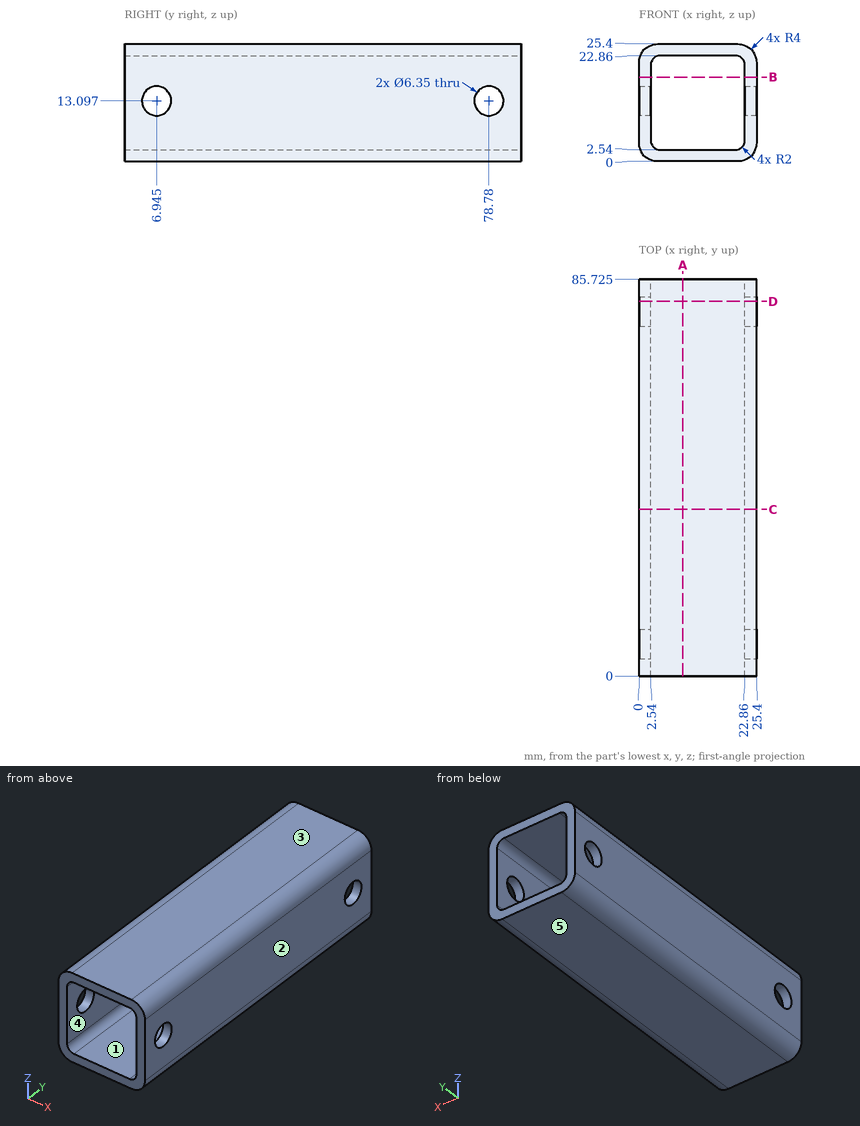
The drawing under review shows one solid part. Ordinate dimensions are in mm from its lowest x, y, z. A direction names the side the tool comes from. Round coordinates to 2 decimals unless told otherwise and drop trailing zeros. Write each loop counter-clockwise with the first axis right and the second up, starting at its lowest first coordinate (ties: lowest second). Pieces come first, ordered by that corner, then holes. Notation, with made-up numbers: (14, 12) -> (67, 12) arc R19 cw to (67, 27) -> close; hole circle Ø3 at (51, -8.5). An arc over 180 degrees is marked (long way). Put each result on its own line as item: value.
Q1. Machinability: for the marked faces 4 and 5, which of the approach directions +Z, -Z, +X, -X, +Y, -Y give a long, thin tool a straight path to every point of the face, cutting with its end or side? Answer none if there is none.
Determined:
face 4: +Y, -Y
face 5: -Z, +X, -X, +Y, -Y
Q2. Consider section D-D on y = 81. State the section outline as (x, z) points, and give its area (3 significant figures).
Determined:
outline: (0, 4) arc R4 ccw to (4, 0) -> (21.4, 0) arc R4 ccw to (25.4, 4) -> (25.4, 10.83) -> (22.86, 10.83) -> (22.86, 4.54) arc R2 cw to (20.86, 2.54) -> (4.54, 2.54) arc R2 cw to (2.54, 4.54) -> (2.54, 10.83) -> (0, 10.83) -> close; (0, 15.37) -> (2.54, 15.37) -> (2.54, 20.86) arc R2 cw to (4.54, 22.86) -> (20.86, 22.86) arc R2 cw to (22.86, 20.86) -> (22.86, 15.37) -> (25.4, 15.37) -> (25.4, 21.4) arc R4 ccw to (21.4, 25.4) -> (4, 25.4) arc R4 ccw to (0, 21.4) -> close
area: 199 mm^2
Q3. Consider section C-C on y = 36. State the section outline as (x, z) points, and give its area (3 significant figures).
Determined:
outline: (0, 4) arc R4 ccw to (4, 0) -> (21.4, 0) arc R4 ccw to (25.4, 4) -> (25.4, 21.4) arc R4 ccw to (21.4, 25.4) -> (4, 25.4) arc R4 ccw to (0, 21.4) -> close; hole (2.54, 4.54) arc R2 ccw to (4.54, 2.54) -> (20.86, 2.54) arc R2 ccw to (22.86, 4.54) -> (22.86, 20.86) arc R2 ccw to (20.86, 22.86) -> (4.54, 22.86) arc R2 ccw to (2.54, 20.86) -> close
area: 222 mm^2
Q4. Consider section B-B on z = 18.25. State the section outline as (x, y) points (1 decimal).
Determined:
outline: (0, 0) -> (2.5, 0) -> (2.5, 85.7) -> (0, 85.7) -> close; (22.9, 0) -> (25.4, 0) -> (25.4, 85.7) -> (22.9, 85.7) -> close
Q5. To check wall thickness, follow L1, parallel to X at y = 79, z = 6.5; L2, parallel to X at y = 56, z = 22 (1 decimal). State the ranges of each line that lie inside material, in increasing order. Write a range as [from, to].
Determined:
L1: x = [0, 2.54], [22.86, 25.4]
L2: x = [0, 2.9], [22.5, 25.4]
Q6. Clearance check with a flat-ended pin moving along its axis: pin 1 Ø3 at (x, z) = (14, 5.5) entering from -Y. State where the tip first meets the part, or that it passes through.
Determined:
pin 1: passes through
Q7. The part is to be moulded in two halves that separate along X. For the marked faces 1, 2 and 3, say which applies: released by +X, released by -X, zero draft, split by the parting line, or undercut.
Determined:
face 1: undercut
face 2: released by +X
face 3: zero draft
Q8. Consider section A-A on x = 9.5. State the section outline as (y, z) points (1 decimal).
Determined:
outline: (0, 0) -> (85.7, 0) -> (85.7, 2.5) -> (0, 2.5) -> close; (0, 22.9) -> (85.7, 22.9) -> (85.7, 25.4) -> (0, 25.4) -> close
